from build123d import *

# Parameters (mm, degrees)
F0_W     = 7
F0_H     = 50
F1_DEPTH = 20
F2_R     = 5
F3_W     = 20
F3_H     = 37.745
F4_DEPTH = 1
F5_SIZE2 = 15
F5_SIZE  = 6
F6_R     = 3.25
F7_DEPTH = 25
F8_SIZE  = 5


with BuildPart() as f1:
    # F0 (on Front) → F1 (new body)
    with BuildSketch(Plane.XZ):
        Rectangle(F0_W, F0_H)
    extrude(amount=F1_DEPTH)

    # F2
    f2_edges = [f1.edges().sort_by_distance(p)[0] for p in [
        (-3.5, -10, -25),
    ]]
    fillet(f2_edges, radius=F2_R)

    # F3 (on face) → F4 (cut)
    with BuildSketch(Plane(origin=(-3.5, 0, 0), x_dir=(0, -1, 0), z_dir=(-1, 0, 0))):
        with Locations((10, -1.1275)):
            Rectangle(F3_W, F3_H)
    extrude(amount=-F4_DEPTH, mode=Mode.SUBTRACT)

    # F5
    f5_edges = [f1.edges().sort_by_distance(p)[0] for p in [
        (3.5, -10, 25),
    ]]
    chamfer(f5_edges, length=F5_SIZE, length2=F5_SIZE2)

    # F6 (on face) → F7 (cut)
    with BuildSketch(Plane.YZ.offset(3.5)):
        with Locations((-10, 0)):
            Circle(F6_R)
    extrude(amount=-F7_DEPTH, mode=Mode.SUBTRACT)

    # F8
    f8_edges = [f1.edges().sort_by_distance(p)[0] for p in [
        (3.5, -20, -7.5),
        (3.5, 0, -7.5),
    ]]
    chamfer(f8_edges, length=F8_SIZE)


solid = f1.part
Source: CAD feature listing. Evaluate the final solid. Frame: model axes, mm. A direction names the side the tool comes from. Coordinates: 2 decimals unless noted, no trailing zeros. Loops run counter-clockwise (first coordinate to the right, second up) from the corner with the lowest first, then second, coordinate; pieces in that order, holes last. Notation, with made-up numbers: (-11.75, -35.5) - (7.25, -35.5) arc R13 cw to (7.25, -23.5) - close; hole circle Ø11 at (59, 21). An arc over 180 degrees is marked (long way). One line per item, written item: value. Start each with the question number.
1. Mould query, pull axis Z, two halves, no side actions, for faces 3 (the flat face through (2, -10, -25)), 4 (the flat face through (-3, -10, 25)), 5 (the flat face through (-3, -10, -20)), 6 (the flat face through (-2, 0, 1)). Classes: pulls with the +Z half, pulls with the -Z half, needs draft (parallel to the pull), parting line crosses it, or undercut.
2. Contact query for flat-ended pins moving along their axis: P1, Ø0.8, axis at x = -3, y = -11.5, coming from the -Z side; P2, Ø2, axis at x = 1, y = -18, coming from the +Z side; P3, Ø12, axis at y = -8.5, z = -7, coming from the -X side. Output: stop coordinate, or through.
3. Set-up query: faces 1 (the cylindrical face through (0.542, -13.247, 0.143)), 2 (the flat face through (-3, -10, 17.745)). Return all of +Z, -Z, +X, -X, +Y, -Y with unobstructed straight access to the full face (end or side cutting, diameter ignored); none if empty.
4. Section C-C (y = -16.5). Return the cut outline in (x, z) (3 decimals), and give its area (3 significant figures).
5. Ray query, L1, parallel to X at y = -14, z = -18; L2, parallel to Z at x = -3, y = -3.25 (3 decimals); L3, parallel to Y at x = -0.25, z = 2. Return the intervals inside material, ascending.
6. Section A-A (y = -10). Return the cut outline in (x, z) (3 decimals).
7. Section D-D (x = -0.5). Return the cut outline in (y, z).
8. Section B-B (z = 0). Return the cut outline in (x, y), and give its area (3 significant figures).
Verdict:
1. face 3: pulls with the -Z half
1. face 4: pulls with the +Z half
1. face 5: undercut
1. face 6: needs draft
2. P1: stops at z = -22.86
2. P2: stops at z = 18.75
2. P3: stops at x = -2.5
3. face 1: +X, -X
3. face 2: -X, +Y, -Y
4. outline: (-3.5, -20) arc R5 ccw to (1.5, -25) - (2, -25) - (2, 13.75) - (-2.5, 25) - (-3.5, 25) - (-3.5, 17.745) - (-2.5, 17.745) - (-2.5, -20) - close
4. area: 207 mm2
5. L1: x = -2.5 to 3.5
5. L2: z = -22.179 to -20, 17.745 to 25
5. L3: y = -18.75 to -12.56, -7.44 to -1.25
6. outline: (-3.5, -20) arc R5 ccw to (1.5, -25) - (3.5, -25) - (3.5, -3.25) - (-2.5, -3.25) - (-2.5, -20) - close; (-3.5, 17.745) - (-2.5, 17.745) - (-2.5, 3.25) - (3.5, 3.25) - (3.5, 10) - (-2.5, 25) - (-3.5, 25) - close
7. outline: (-19, -24.58) - (-1, -24.58) - (-1, 20) - (-19, 20) - close; hole circle Ø6.5 at (-10, 0)
8. outline: (-2.5, -20) - (-1.5, -20) - (3.5, -15) - (3.5, -13.25) - (-2.5, -13.25) - close; (-2.5, -6.75) - (3.5, -6.75) - (3.5, -5) - (-1.5, 0) - (-2.5, 0) - close
8. area: 56.0 mm2
